from build123d import *

# Parameters (mm, degrees)
EXTRUDE1_DEPTH = 40
EXTRUDE2_REACH = 42
SKETCH2_R      = 1.5
EXTRUDE3_REACH = 42
SKETCH3_R      = 1.5
CHAMFER1_SIZE  = 2


with BuildPart() as part:
    # Sketch1 → Extrude1 (new body)
    with BuildSketch(Plane(origin=(0, 0, 0), x_dir=(0, 0, -1), z_dir=(1, 0, 0))):
        Polygon((0, 0), (0, 38), (2, 38), (2, -2), (-38, -2), (-38, 0), align=None)
    extrude(amount=EXTRUDE1_DEPTH)

    # Sketch2 → Extrude2 (cut, up to next)
    with BuildSketch(Plane(origin=(0, -2, 0), x_dir=(-1, 0, 0), z_dir=(0, -1, 0)), mode=Mode.PRIVATE) as extrude2_sk1:
        with Locations((-32.5, -23.75)):
            Circle(SKETCH2_R)
    extrude2_tool1 = extrude(extrude2_sk1.sketch, amount=-EXTRUDE2_REACH, mode=Mode.PRIVATE) & part.part
    add(extrude2_tool1.solids().sort_by_distance((32.5, -2, 23.75))[0], mode=Mode.SUBTRACT)
    # Sketch2 → Extrude2 (cut, up to next)
    with BuildSketch(Plane(origin=(0, -2, 0), x_dir=(-1, 0, 0), z_dir=(0, -1, 0)), mode=Mode.PRIVATE) as extrude2_sk2:
        with Locations((-7.5, -23.75)):
            Circle(SKETCH2_R)
    extrude2_tool2 = extrude(extrude2_sk2.sketch, amount=-EXTRUDE2_REACH, mode=Mode.PRIVATE) & part.part
    add(extrude2_tool2.solids().sort_by_distance((7.5, -2, 23.75))[0], mode=Mode.SUBTRACT)

    # Sketch3 → Extrude3 (cut, up to next)
    with BuildSketch(Plane(origin=(0, 0, -2), x_dir=(-1, 0, 0), z_dir=(0, 0, -1)), mode=Mode.PRIVATE) as extrude3_sk1:
        with Locations((-10, 31.9)):
            Circle(SKETCH3_R)
    extrude3_tool1 = extrude(extrude3_sk1.sketch, amount=-EXTRUDE3_REACH, mode=Mode.PRIVATE) & part.part
    add(extrude3_tool1.solids().sort_by_distance((10, 31.9, -2))[0], mode=Mode.SUBTRACT)
    # Sketch3 → Extrude3 (cut, up to next)
    with BuildSketch(Plane(origin=(0, 0, -2), x_dir=(-1, 0, 0), z_dir=(0, 0, -1)), mode=Mode.PRIVATE) as extrude3_sk2:
        with Locations((-30, 31.9)):
            Circle(SKETCH3_R)
    extrude3_tool2 = extrude(extrude3_sk2.sketch, amount=-EXTRUDE3_REACH, mode=Mode.PRIVATE) & part.part
    add(extrude3_tool2.solids().sort_by_distance((30, 31.9, -2))[0], mode=Mode.SUBTRACT)
    # Sketch3 → Extrude3 (cut, up to next)
    with BuildSketch(Plane(origin=(0, 0, -2), x_dir=(-1, 0, 0), z_dir=(0, 0, -1)), mode=Mode.PRIVATE) as extrude3_sk3:
        with Locations((-30, 11.9)):
            Circle(SKETCH3_R)
    extrude3_tool3 = extrude(extrude3_sk3.sketch, amount=-EXTRUDE3_REACH, mode=Mode.PRIVATE) & part.part
    add(extrude3_tool3.solids().sort_by_distance((30, 11.9, -2))[0], mode=Mode.SUBTRACT)
    # Sketch3 → Extrude3 (cut, up to next)
    with BuildSketch(Plane(origin=(0, 0, -2), x_dir=(-1, 0, 0), z_dir=(0, 0, -1)), mode=Mode.PRIVATE) as extrude3_sk4:
        with Locations((-10, 11.9)):
            Circle(SKETCH3_R)
    extrude3_tool4 = extrude(extrude3_sk4.sketch, amount=-EXTRUDE3_REACH, mode=Mode.PRIVATE) & part.part
    add(extrude3_tool4.solids().sort_by_distance((10, 11.9, -2))[0], mode=Mode.SUBTRACT)

    # Chamfer1
    chamfer1_edges = [part.edges().sort_by_distance(p)[0] for p in [
        (40, 38, -1),
        (0, 38, -1),
        (40, -1, 38),
        (0, -1, 38),
    ]]
    chamfer(chamfer1_edges, length=CHAMFER1_SIZE)


solid = part.part
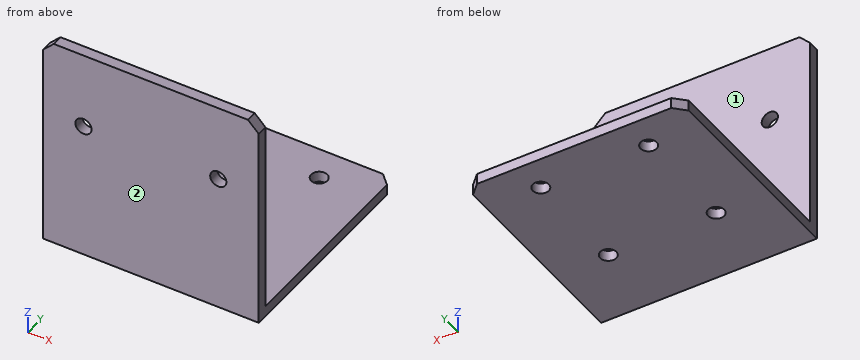
Input: part model. Units: mm. Frame: model coordinates. Face numbers are marked on the shaded views. A direction names the side the tool comes from. Round coordinates to 2 decimals unless told otherwise and drop trailing zeros. Write each loop counter-clockwise with the first axis right and the second up, starting at its lowest first coordinate (ties: lowest second). Pieces come first, ordered by that corner, then holes.
1) Contact query for flat-ended pins moving along their axis: P1, Ø1.5, axis at x = 22.5, y = 33.5, coming from the +Z side; P2, Ø3, axis at x = 5, z = 13, coming from the +Y side. Output: stop coordinate, or through.
2) Cut plane C-C (y = 11.9). Return the cut outline in (x, z).
3) Cut plane A-A (z = 23.75). Return the cut outline in (x, y).
4) Ray query, L1, parallel to Y at x = 30, z = -0.65; L2, parallel to Z at x = 15.5, y = 24. Return the intervals inside material, ascending.
5) Cut plane D-D (x = 10). Return the cut outline in (y, z), then the cut area to 3 significant figures.
6) Cut plane B-B (x = 32.5). Return the cut outline in (y, z), then the cut area to 3 significant figures.
7) Reachability of the marked faces 1 and 2 from +Z, -Z, +X, -X, +Y, -Y: full face, straight path, thin tool, end or side. Return the list, or none.
Geometry says:
1. P1: stops at z = 0
1. P2: stops at y = 0
2. outline: (0, -2) - (8.5, -2) - (8.5, 0) - (0, 0) - close; (11.5, -2) - (28.5, -2) - (28.5, 0) - (11.5, 0) - close; (31.5, -2) - (40, -2) - (40, 0) - (31.5, 0) - close
3. outline: (0, -2) - (6, -2) - (6, 0) - (0, 0) - close; (9, -2) - (31, -2) - (31, 0) - (9, 0) - close; (34, -2) - (40, -2) - (40, 0) - (34, 0) - close
4. L1: y = -2 to 10.4, 13.4 to 30.4, 33.4 to 38
4. L2: z = -2 to 0
5. outline: (-2, -2) - (10.4, -2) - (10.4, 0) - (0, 0) - (0, 38) - (-2, 38) - close; (13.4, -2) - (30.4, -2) - (30.4, 0) - (13.4, 0) - close; (33.4, -2) - (38, -2) - (38, 0) - (33.4, 0) - close
5. area: 144 mm2
6. outline: (-2, -2) - (38, -2) - (38, 0) - (0, 0) - (0, 22.25) - (-2, 22.25) - close; (-2, 25.25) - (0, 25.25) - (0, 38) - (-2, 38) - close
6. area: 150 mm2
7. face 1: +Z, +X, -X, +Y
7. face 2: +Z, -Z, +X, -X, -Y
